Model file for the job. Use its own axes, mm. Face numbers are marked on the shaded views. Give positions to 0.01 mm unless a question says otherwise; leave off trailing zeros. Write each loop counter-clockwise with the first axis right and the second up, starting at its lowest first coordinate (ties: lowest second). Pieces come first, ordered by that corner, then holes. Notation, with made-up numbers: (58, 13.25) - (76, 13.25) arc R22 cw to (76, 46.25) - close; hole circle Ø6 at (26.25, 63.25). An arc over 180 degrees is marked (long way). Use a Markdown table: item, result. Add a question column.
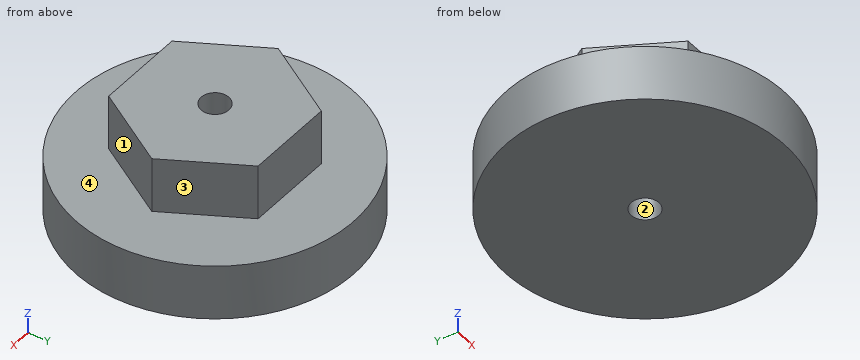
```python
from build123d import *

# Parameters (mm, degrees)
SKETCH1_R           = 25.139311184
BOSS_EXTRUDE1_DEPTH = 10
SKETCH1_3_R         = 2.5
BOSS_EXTRUDE2_DEPTH = 20


with BuildPart() as part:
    # Sketch1 → Boss-Extrude1 (new body)
    with BuildSketch(Plane.XY):
        Circle(SKETCH1_R)
        Polygon((15.612098952, -0.280612845), (8.049067329, 13.380167876), (-7.563031623, 13.660780721), (-15.612098952, 0.280612845), (-8.049067329, -13.380167876), (7.563031623, -13.660780721), align=None, mode=Mode.SUBTRACT)
    extrude(amount=BOSS_EXTRUDE1_DEPTH)

    # Sketch1_3 → Boss-Extrude2 (add)
    with BuildSketch(Plane.XY):
        Polygon((7.563031623, -13.660780721), (15.612098952, -0.280612845), (8.049067329, 13.380167876), (-7.563031623, 13.660780721), (-15.612098952, 0.280612845), (-8.049067329, -13.380167876), align=None)
        Circle(SKETCH1_3_R, mode=Mode.SUBTRACT)
    extrude(amount=BOSS_EXTRUDE2_DEPTH)


solid = part.part
```
(1) Band-saw the part on A-A (z = 17). Write the cut outline in (x, y), then the cut area to 3 significant figures.
(2) Flat gauge pins, fed straight in: pin 1 (3 mm diameter, centred on x = 0, y = 0, fed in from -Z); pin 2 (1 mm diameter, centred on x = -20, y = 15.5, fed in from +Z); pin 3 (3 mm diameter, centred on x = -3.5, y = -3.5, fed in from -Z); pin 4 (5 mm diameter, centred on y = 15, z = 3, fed in from -X). Where does each tip first touch, or does it go through?
(3) Two-plate mould, pull along Y, no slides. Class the marked faces 1, 2, 3 and 4: +Y half, -Y half, draft (parallel to the pull), parting line (faces both ways), or undercut.
(4) Probe probe 1 along Y at (x, z) = (0, 6); probe 2 along Z at (x, y) = (15.5, -17.5); probe 3 along Y at (x, z) = (0, 15.25). List the from-to ranges inside material, lowest first. Write a range as [from, to].
(5) Band-saw the part on C-C (x = 6). Write the cut outline in (y, z).
(6) Band-saw the part on D-D (y = -7.5). Write the cut outline in (x, z).
(7) Band-saw the part on B-B (x = 0). Write the cut outline in (y, z).
Model answer:
| question | item | result |
|---|---|---|
| 1 | outline | (-15.61, 0.28) - (-8.05, -13.38) - (7.56, -13.66) - (15.61, -0.28) - (8.05, 13.38) - (-7.56, 13.66) - close; hole circle Ø5 at (0, 0) |
| 1 | area | 614 mm^2 |
| 2 | pin 1 | passes through |
| 2 | pin 2 | stops at z = 10 |
| 2 | pin 3 | stops at z = 0 |
| 2 | pin 4 | stops at x = -21.81 |
| 3 | face 1 | -Y half |
| 3 | face 2 | undercut |
| 3 | face 3 | +Y half |
| 3 | face 4 | draft |
| 4 | probe 1 | y = [-25.14, -2.5], [2.5, 25.14] |
| 4 | probe 2 | z = [0, 10] |
| 4 | probe 3 | y = [-13.52, -2.5], [2.5, 13.52] |
| 5 | outline | (-24.41, 0) - (24.41, 0) - (24.41, 10) - (13.42, 10) - (13.42, 20) - (-13.63, 20) - (-13.63, 10) - (-24.41, 10) - close |
| 6 | outline | (-23.99, 0) - (23.99, 0) - (23.99, 10) - (11.27, 10) - (11.27, 20) - (-11.3, 20) - (-11.3, 10) - (-23.99, 10) - close |
| 7 | outline | (-25.14, 0) - (-2.5, 0) - (-2.5, 20) - (-13.52, 20) - (-13.52, 10) - (-25.14, 10) - close; (2.5, 0) - (25.14, 0) - (25.14, 10) - (13.52, 10) - (13.52, 20) - (2.5, 20) - close |
